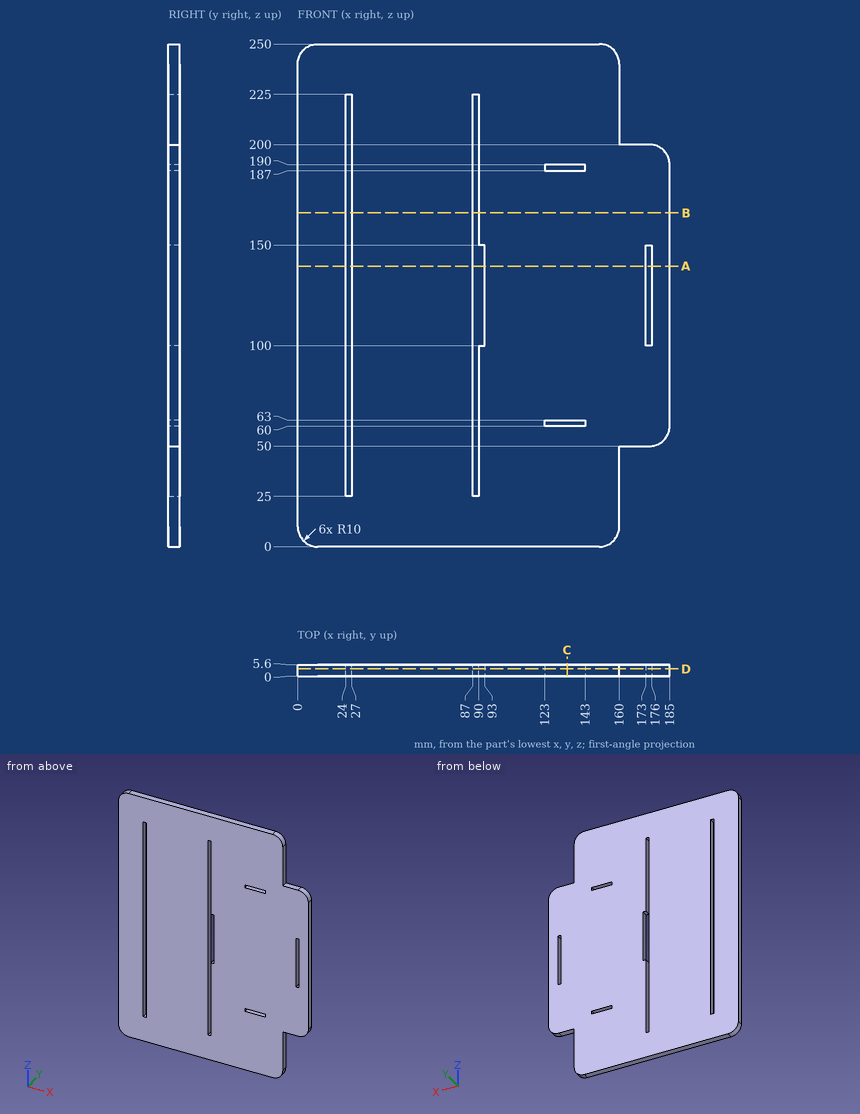
Check sheet for the drawn part. Datum: minimum x, y, z corner. Units: mm. Give positions to 0.01 mm unless a question says otherwise; leave off trailing zeros. Order: outer loops, then holes, each group sorted by start corner. A loop starts at its lowest first (then second) coordinate and runs counter-clockwise, first axis right, second up. Notation, with made-up numbers: (38, 19.25) - (44, 19.25) arc R14 ccw to (44, 31.25) - close; hole circle Ø5 at (-6, 58.25). An arc over 180 degrees is marked (long way). Answer in a Markdown table with one row per item. Add a question column.
Q1. Cross-section at B-B, the plane z = 166. Enter the section's corners in (x, y).
Q2. Gauge pin test, flat ends, axial feed: pin 1 (1.7 mm diameter, centred on x = 167, y = 2.5, fed in from -Z); pin 2 (1.7 mm diameter, centred on x = 171, y = 3.5, fed in from +Z); pin 3 (3 mm diameter, centred on y = 2.5, z = 220.5, fed in from +X). Record the tip position at first contact, or that the pin passes through.
Q3. Cross-section at A-A, the plane z = 139.5. Enter the section's corners in (x, y).
Q4. Cross-section at C-C, the plane x = 134. Enter the section's corners in (y, z).
Q5. Cross-section at D-D, the plane y = 3.6. Count the separate pieces of the cut face and the enclosed holes in it, then the cut area to 3 significant figures.
Q6. Material ranges on probe 1 along X at (y, z) = (0.8, 102); probe 2 along X at (y, z) = (3.4, 30); probe 3 along Z at (x, y) = (138.5, 3.55), recorded low to high. Write a range as from..to.
Check values:
| question | item | result |
|---|---|---|
| 1 | outline | (0, 0) - (24, 0) - (24, 5.6) - (0, 5.6) - close; (27, 0) - (87, 0) - (87, 5.6) - (27, 5.6) - close; (90, 0) - (185, 0) - (185, 5.6) - (90, 5.6) - close |
| 2 | pin 1 | stops at z = 50 |
| 2 | pin 2 | stops at z = 200 |
| 2 | pin 3 | stops at x = 160 |
| 3 | outline | (0, 0) - (24, 0) - (24, 5.6) - (0, 5.6) - close; (27, 0) - (87, 0) - (87, 5.6) - (27, 5.6) - close; (93, 0) - (173, 0) - (173, 5.6) - (93, 5.6) - close; (176, 0) - (185, 0) - (185, 5.6) - (176, 5.6) - close |
| 4 | outline | (0, 0) - (5.6, 0) - (5.6, 60) - (0, 60) - close; (0, 63) - (5.6, 63) - (5.6, 187) - (0, 187) - close; (0, 190) - (5.6, 190) - (5.6, 250) - (0, 250) - close |
| 5 | separate pieces | 1 |
| 5 | enclosed holes | 5 |
| 5 | area | 42,000 mm^2 |
| 6 | probe 1 | x = 0..24, 27..87, 93..173, 176..185 |
| 6 | probe 2 | x = 0..24, 27..87, 90..160 |
| 6 | probe 3 | z = 0..60, 63..187, 190..250 |
